from build123d import *

# Parameters (mm, degrees)
SKETCH_1_R          = 2.1
EXTRUDE_1_DEPTH     = 7.5
SKETCH_5_R          = 3.4
EXTRUDE_2_DEPTH     = 10
SKETCH_7_R          = 3.1
SKETCH_6_R          = 3.4
SKETCH_8_R          = 1.25
CUT_EXTRUDE_1_DEPTH = 21.27831367


with BuildPart() as part:
    # 草图1 → 凸台-拉伸1 (new body)
    with BuildSketch(Plane(origin=(0, 0, 0), x_dir=(1, 0, 0), z_dir=(0, 1, 0))):
        with Locations(Location((0, 0, 0), (0, 0, 270))):
            Circle(SKETCH_1_R)
    extrude(amount=EXTRUDE_1_DEPTH)

    # 放样1: read off the stored shape, not the designer's step
    # 放样1: loft between two sections, ruled curve by curve
    loft_1_from = [
        Edge.make_bspline([(-3.388135234, 7.5, 0.283795064), (-3.955725362, 7.5, -6.492475403), (2.820545105, 7.5, -7.060065531), (3.388135234, 7.5, -0.283795064), (3.955725362, 7.5, 6.492475403), (-2.820545105, 7.5, 7.060065531), (-3.388135234, 7.5, 0.283795064)], [0, 0, 0, 0, 0.5, 0.5, 0.5, 1, 1, 1, 1], 3, [1, 0.333333333, 0.333333333, 1, 0.333333333, 0.333333333, 1]),
    ]
    loft_1_to = [
        Edge.make_bspline([(-1.894481315, 3.5, 0.906057696), (-3.706596707, 3.5, -2.882904933), (0.082365923, 3.5, -4.695020325), (1.894481315, 3.5, -0.906057696), (3.706596707, 3.5, 2.882904933), (-0.082365923, 3.5, 4.695020325), (-1.894481315, 3.5, 0.906057696)], [0, 0, 0, 0, 0.5, 0.5, 0.5, 1, 1, 1, 1], 3, [1, 0.333333333, 0.333333333, 1, 0.333333333, 0.333333333, 1]),
    ]
    loft_1 = Solid(Shell([*[Face.make_surface_from_curves(loft_1_from[k], loft_1_to[k]) for k in range(1)], Face(Wire(loft_1_from)), Face(Wire(loft_1_to))]))
    add(loft_1)

    # 草图5 → 凸台-拉伸2 (add)
    with BuildSketch(Plane(origin=(0, 7.5, 0), x_dir=(1, 0, 0), z_dir=(0, 1, 0))):
        with Locations(Location((0, 0, 0), (0, 0, 270))):
            Circle(SKETCH_5_R)
    extrude(amount=EXTRUDE_2_DEPTH)

    # 草图7 → 放样2 section 0
    with BuildSketch(Plane(origin=(0, 19.7, 0), x_dir=(1, 0, 0), z_dir=(0, 1, 0))):
        Circle(SKETCH_7_R)
    # 草图6 → 放样2 section 1
    with BuildSketch(Plane(origin=(0, 17.5, 0), x_dir=(1, 0, 0), z_dir=(0, 1, 0))):
        Circle(SKETCH_6_R)
    loft()

    # 草图8 → 切除-拉伸1 (cut, through all)
    with BuildSketch(Plane(origin=(0, 19.7, 0), x_dir=(1, 0, 0), z_dir=(0, 1, 0))):
        with Locations(Location((0, 0, 0), (0, 0, 270))):
            Circle(SKETCH_8_R)
    extrude(amount=-CUT_EXTRUDE_1_DEPTH, mode=Mode.SUBTRACT)


solid = part.part
Input: part model. Units: mm. Frame: model coordinates. A direction names the side the tool comes from. Give positions to 0.01 mm unless a question says otherwise; leave off trailing zeros. Loops run counter-clockwise (first coordinate to the right, second up) from the corner with the lowest first, then second, coordinate; pieces in that order, holes last. Notation, with made-up numbers: M 89.25,-34.5 L 97.25,-34.5 A26 cw 97.25,-11.5 Z; hole C 12.25,79 d4. An arc over 180 degrees is marked long. Use one line per item in the form item = value.
1. First-contact query: pin 1 (1 mm diameter, centred on y = 6, z = 0, fed in from +X); pin 2 (3 mm diameter, centred on x = -0.5, y = 4, fed in from +Z); pin 3 (1.5 mm diameter, centred on y = 15.5, z = -2, fed in from +X). Flat tips, straight axial feed; report the tip coordinate or a pass-through.
Numbers:
pin_1 = 3.05
pin_2 = 2.69
pin_3 = 3.16
2. Line query: L1, parallel to X at y = 11.5, z = 0; L2, parallel to Z at x = -0.5, y = 18.75; L3, parallel to X at y = 2.75, z = 0.5. Output: solid intervals per line, ascending.
Numbers:
L1 = -3.4 to -1.25, 1.25 to 3.4
L2 = -3.19 to -1.15, 1.15 to 3.19
L3 = -2.04 to -1.15, 1.15 to 2.04
3. Pull-direction query (X, two-part tool) for faces 1 (the face through (-1.22, 9.99, -0.27)), 2 (the face through (-0.41, 19.07, -3.16)), 3 (the face through (1, 19.7, 1)); classes: released by +X, released by -X, zero draft, split by the parting line, or undercut.
Numbers:
face_1 = undercut
face_2 = split by the parting line
face_3 = zero draft
4. Reachability of faces 4 (the face through (-3.32, 12.43, -0.74)), 5 (the face through (0.631, 1.726, 2.003)) from +Z, -Z, +X, -X, +Y, -Y: full face, straight path, thin tool, end or side. Return the list, or none.
Numbers:
face_4 = +Y, -Y
face_5 = -Y
5. Section query A-A, the plane y = 13.75. Return the cut outline in (x, z), and give its area (3 significant figures).
Numbers:
outline = C 0,0 d6.8; hole C 0,0 d2.5
area = 31.4 mm²
